Source: CAD feature listing. Evaluate the final solid. Frame: model axes, mm. Give positions to 0.01 mm unless a question says otherwise; leave off trailing zeros. Loops run counter-clockwise (first coordinate to the right, second up) from the corner with the lowest first, then second, coordinate; pieces in that order, holes last.
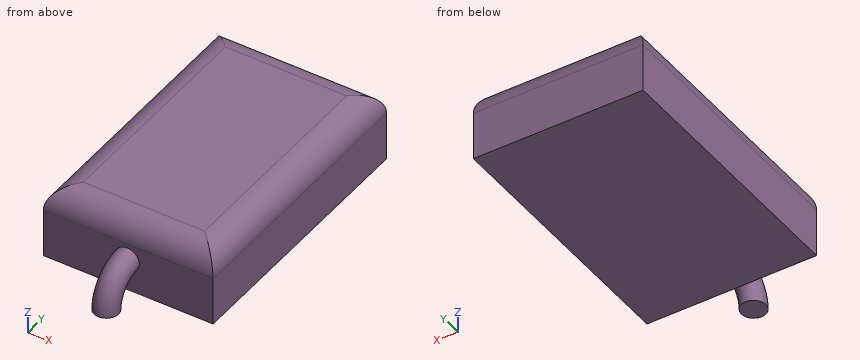
from build123d import *

# Parameters (mm, degrees)
F0_W     = 35.56
F0_H     = 55.88
F1_DEPTH = 15.24
F2_R     = 5.08
F3_R     = 2.549678
F4_ANGLE = 90


with BuildPart() as f1:
    # F0 (on Top) → F1 (new body)
    with BuildSketch(Plane.XY):
        with Locations((-27.240339, 1.234332)):
            Rectangle(F0_W, F0_H)
    extrude(amount=F1_DEPTH)

    # F2
    f2_edges = [f1.edges().sort_by_distance(p)[0] for p in [
        (-27.240339, 29.174332, 15.24),
        (-45.020339, 1.234332, 15.24),
        (-27.240339, -26.705668, 15.24),
        (-9.460339, 1.234332, 15.24),
    ]]
    fillet(f2_edges, radius=F2_R)

    # F3 (on face) → F4 (revolve)
    with BuildSketch(Plane.XZ.offset(26.705668)):
        with Locations((-27.447378, 6.727298)):
            Circle(F3_R)
    revolve(axis=Axis((-27.240339, -26.705668, 0), (1, 0, 0)), revolution_arc=F4_ANGLE)


solid = f1.part
1) Cut plane D-D (x = -29). Return loops of the section in (y, z), and give its area (3 significant figures).
Checks:
outline: (-35.46, 0) - (-31.41, 0) arc R4.7 cw to (-26.71, 4.7) - (-26.71, 0) - (29.17, 0) - (29.17, 10.16) arc R5.08 ccw to (24.09, 15.24) - (-21.63, 15.24) arc R5.08 ccw to (-26.71, 10.16) - (-26.71, 8.75) arc R8.75 ccw to start
area: 883 mm2
2) Cut plane B-B (y = 14.5). Return loops of the section in (x, z).
Checks:
outline: (-45.02, 0) - (-9.46, 0) - (-9.46, 10.16) arc R5.08 ccw to (-14.54, 15.24) - (-39.94, 15.24) arc R5.08 ccw to (-45.02, 10.16) - close
3) Cut plane A-A (x = -35.5). Return loops of the section in (y, z), and give its area (3 significant figures).
Checks:
outline: (-26.71, 0) - (29.17, 0) - (29.17, 10.16) arc R5.08 ccw to (24.09, 15.24) - (-21.63, 15.24) arc R5.08 ccw to (-26.71, 10.16) - close
area: 841 mm2
4) Contact query for flat-ended pins moving along their axis: P1, Ø1, axis at x = -28, z = 10.5, coming from the -Y side; P2, Ø2, axis at x = -25.5, z = 3, coming from the -Y side. Output: stop coordinate, or through.
Checks:
P1: stops at y = -26.71
P2: stops at y = -35.39
5) Cut plane C-C (z = 12.75). Return loops of the section in (x, y), and give its area (3 significant figures).
Checks:
outline: (-44.31, -26) - (-10.17, -26) - (-10.17, 28.46) - (-44.31, 28.46) - close
area: 1,860 mm2
6) Ray query, probe 1 along X at (y, z) = (-10.5, 10.5); probe 2 along Y at (x, z) = (-42, 1.5); probe 3 along Y at (x, z) = (-34.5, 10.75). Return the intervals inside material, ascending.
Checks:
probe 1: x = -45.01 to -9.47
probe 2: y = -26.71 to 29.17
probe 3: y = -26.67 to 29.14
